```python
from build123d import *

# Parameters (mm, degrees)
SKETCH1_W           = 50
SKETCH1_H           = 30
BOSS_EXTRUDE1_DEPTH = 15
SKETCH2_R           = 2.45
CUT_EXTRUDE1_DEPTH  = 31
SKETCH3_R           = 1.25
CUT_EXTRUDE2_DEPTH  = 16


with BuildPart() as part:
    # Sketch1 → Boss-Extrude1 (new body)
    with BuildSketch(Plane(origin=(0, 0, 0), x_dir=(1, 0, 0), z_dir=(0, 1, 0))):
        with Locations((25, 15)):
            Rectangle(SKETCH1_W, SKETCH1_H)
    extrude(amount=BOSS_EXTRUDE1_DEPTH)

    # Sketch2 → Cut-Extrude1 (cut, through all)
    with BuildSketch(Plane.XY):
        with Locations((35, 7.5)):
            Circle(SKETCH2_R)
        with Locations((15, 7.5)):
            Circle(SKETCH2_R)
    extrude(amount=-CUT_EXTRUDE1_DEPTH, mode=Mode.SUBTRACT)

    # Sketch3 → Cut-Extrude2 (cut, through all)
    with BuildSketch(Plane(origin=(0, 15, 0), x_dir=(1, 0, 0), z_dir=(0, 1, 0))):
        with Locations((20, 13.518993942)):
            Circle(SKETCH3_R)
    extrude(amount=-CUT_EXTRUDE2_DEPTH, mode=Mode.SUBTRACT)


solid = part.part
```
Can you work these out from the model? Positions are in its coordinate system, mm. Coordinates: 2 decimals unless noted, no trailing zeros. Loops run counter-clockwise (first coordinate to the right, second up) from the corner with the lowest first, then second, coordinate; pieces in that order, holes last.
1) I need wall thicknesses on probe 1 along Y at (x, z) = (35, -7); probe 2 along Z at (x, y) = (20, 8); probe 3 along X at (y, z) = (7.75, -22.5). Which ranges of each line are inside material? Lowest first, please.
2) Imagine slicing it at D-D on x = 15. List the corners of the cut face in (y, z) for me, plus the area to 3 significant figures.
3) Imagine slicing it at A-A on x = 20. List the corners of the cut face in (y, z) for me, plus the area to 4 significant figures.
4) Thinking about a two-plate mould opening in Y: for faces 1 (the flat face through (25, 15, -15)), 2 (the flat face through (0, 7, -15)), 3 (the cylindrical face through (12.552, 7.608, -14.79)), which applies, pulls with the +Y half, pulls with the -Y half, needs draft (parallel to the pull), parting line crosses it, or undercut?
5) For pin 1 (2 mm diameter, centred on x = 20, z = -13.52, fed in from +Y), with a flat end and sliding along its axis, tell me the tip position at first contact or that it passes through.
6) Imagine slicing it at C-C on y = 6.25. List the corners of the cut face in (x, z) for me, plus the area to 3 significant figures.
7) Imagine slicing it at B-B on z = -13. List the corners of the cut face in (x, y) for me.
Completed:
1. probe 1: y = 0 to 5.05, 9.95 to 15
1. probe 2: z = -30 to -14.77, -12.27 to 0
1. probe 3: x = 0 to 12.56, 17.44 to 32.56, 37.44 to 50
2. outline: (0, -30) - (5.05, -30) - (5.05, 0) - (0, 0) - close; (9.95, -30) - (15, -30) - (15, 0) - (9.95, 0) - close
2. area: 303 mm2
3. outline: (0, -30) - (15, -30) - (15, -14.77) - (0, -14.77) - close; (0, -12.27) - (15, -12.27) - (15, 0) - (0, 0) - close
3. area: 412.5 mm2
4. face 1: pulls with the +Y half
4. face 2: needs draft
4. face 3: undercut
5. pin 1: passes through
6. outline: (0, -30) - (12.89, -30) - (12.89, 0) - (0, 0) - close; (17.11, -30) - (32.89, -30) - (32.89, 0) - (17.11, 0) - close; (37.11, -30) - (50, -30) - (50, 0) - (37.11, 0) - close; hole circle Ø2.5 at (20, -13.52)
6. area: 1,240 mm2
7. outline: (0, 0) - (18.86, 0) - (18.86, 15) - (0, 15) - close; (21.14, 0) - (50, 0) - (50, 15) - (21.14, 15) - close; hole circle Ø4.9 at (15, 7.5); hole circle Ø4.9 at (35, 7.5)
